```python
from build123d import *

# Parameters (mm, degrees)
SKETCH1_R           = 1.355900406
BOSS_EXTRUDE1_DEPTH = 1.5875
SKETCH3_R           = 1.524
CUT_EXTRUDE1_DEPTH  = 2.5875
SKETCH5_W           = 2.0955
SKETCH5_H           = 13.208
BOSS_EXTRUDE3_DEPTH = 1.5875
CUT_EXTRUDE2_DEPTH  = 2.5875
SKETCH8_R           = 2.4257
CUT_EXTRUDE3_DEPTH  = 2.5875


with BuildPart() as part:
    # Sketch1 → Boss-Extrude1 (new body)
    with BuildSketch(Plane.XY):
        with BuildLine():
            Line((-301.9473, 111.74645), (-305.87795, 115.6771))
            Line((-305.87795, 115.6771), (-316.1078, 115.6771))
            Line((-316.1078, 115.6771), (-316.1078, 128.8851))
            Line((-316.1078, 128.8851), (-305.87795, 128.8851))
            Line((-305.87795, 128.8851), (-301.9473, 132.81575))
            Line((-301.9473, 132.81575), (-301.9473, 150.9704))
            ThreePointArc((-301.9473, 150.9704), (-303.063223164, 153.664476836), (-305.7573, 154.7804))
            Line((-305.7573, 154.7804), (-397.247125, 154.7804))
            ThreePointArc((-397.247125, 154.7804), (-399.946077222, 153.659592612), (-401.0571, 150.956597849))
            Line((-401.0571, 150.956597849), (-401.0571, 148.341))
            Line((-401.0571, 148.341), (-399.1521, 148.341))
            Line((-399.1521, 148.341), (-399.1521, 95.6449))
            Line((-399.1521, 95.6449), (-401.0571, 95.6449))
            Line((-401.0571, 95.6449), (-401.0571, 91.659304166))
            ThreePointArc((-401.0571, 91.659304166), (-399.951018769, 88.947400452), (-397.2472, 87.8217))
            Line((-397.2472, 87.8217), (-378.5565, 87.8217))
            Line((-378.5565, 87.8217), (-368.3165, 91.1883))
            Line((-368.3165, 91.1883), (-315.9973, 91.1883))
            Line((-315.9973, 91.1883), (-305.7573, 87.8217))
            ThreePointArc((-305.7573, 87.8217), (-303.063223164, 88.937623164), (-301.9473, 91.6317))
            Line((-301.9473, 91.6317), (-301.9473, 111.74645))
        make_face()
        with Locations((-305.7573, 91.6317)):
            Circle(SKETCH1_R, mode=Mode.SUBTRACT)
        with Locations((-305.7573, 150.9704)):
            Circle(SKETCH1_R, mode=Mode.SUBTRACT)
        with Locations((-397.247125, 150.9704)):
            Circle(SKETCH1_R, mode=Mode.SUBTRACT)
        with Locations((-397.2472, 91.6317)):
            Circle(SKETCH1_R, mode=Mode.SUBTRACT)
    extrude(amount=BOSS_EXTRUDE1_DEPTH)

    # Sketch3 → Cut-Extrude1 (cut, through all)
    with BuildSketch(Plane.XY.offset(1.5875)):
        with Locations((-397.247125, 150.9704)):
            Circle(SKETCH3_R)
        with Locations((-305.7573, 150.9704)):
            Circle(SKETCH3_R)
        with Locations((-305.7573, 91.6317)):
            Circle(SKETCH3_R)
        with Locations((-397.2472, 91.6317)):
            Circle(SKETCH3_R)
    extrude(amount=-CUT_EXTRUDE1_DEPTH, mode=Mode.SUBTRACT)

    # Sketch5 → Boss-Extrude3 (add)
    with BuildSketch(Plane.XY.offset(1.5875)):
        with Locations((-315.06005, 122.2811)):
            Rectangle(SKETCH5_W, SKETCH5_H)
    extrude(amount=-BOSS_EXTRUDE3_DEPTH)

    # Sketch4 → Cut-Extrude2 (cut, through all)
    with BuildSketch(Plane.XY.offset(1.5875)):
        Polygon((-301.9473, 133.571034757), (-305.87795, 129.6471), (-314.0123, 129.6471), (-314.0123, 113.6451), (-305.87795, 113.6451), (-301.9473, 109.71445), align=None)
    extrude(amount=-CUT_EXTRUDE2_DEPTH, mode=Mode.SUBTRACT)

    # Sketch8 → Cut-Extrude3 (cut, through all)
    with BuildSketch(Plane.XY.offset(1.5875)):
        with Locations((-363.6180125, 150.7799)):
            Circle(SKETCH8_R)
        with Locations((-355.5408125, 150.7799)):
            Circle(SKETCH8_R)
        with Locations((-347.4636125, 150.7799)):
            Circle(SKETCH8_R)
        with Locations((-339.3864125, 150.7799)):
            Circle(SKETCH8_R)
        with Locations((-339.3864125, 142.7027)):
            Circle(SKETCH8_R)
        with Locations((-347.4636125, 142.7027)):
            Circle(SKETCH8_R)
        with Locations((-355.5408125, 142.7027)):
            Circle(SKETCH8_R)
        with Locations((-363.6180125, 142.7027)):
            Circle(SKETCH8_R)
        with Locations((-363.6180125, 95.1888)):
            Circle(SKETCH8_R)
        with Locations((-339.3864125, 95.1888)):
            Circle(SKETCH8_R)
        with Locations((-347.4636125, 95.1888)):
            Circle(SKETCH8_R)
        with Locations((-355.5408125, 95.1888)):
            Circle(SKETCH8_R)
        with Locations((-363.6180125, 103.266)):
            Circle(SKETCH8_R)
        with Locations((-355.5408125, 103.266)):
            Circle(SKETCH8_R)
        with Locations((-347.4636125, 103.266)):
            Circle(SKETCH8_R)
        with Locations((-339.3864125, 103.266)):
            Circle(SKETCH8_R)
    extrude(amount=-CUT_EXTRUDE3_DEPTH, mode=Mode.SUBTRACT)


solid = part.part
```
The model under review builds one solid part; all positions refer to its coordinate system, in mm. A direction names the side the tool comes from. Round coordinates to 2 decimals unless told otherwise and drop trailing zeros. Loops run counter-clockwise (first coordinate to the right, second up) from the corner with the lowest first, then second, coordinate; pieces in that order, holes last.
1) Consider section A-A on x = -339. State the section outline as (y, z) points, then the cut area to 3 significant figures.
Values follow:
outline: (91.19, 0) - (92.79, 0) - (92.79, 1.59) - (91.19, 1.59) - close; (97.58, 0) - (100.87, 0) - (100.87, 1.59) - (97.58, 1.59) - close; (105.66, 0) - (140.31, 0) - (140.31, 1.59) - (105.66, 1.59) - close; (145.1, 0) - (148.39, 0) - (148.39, 1.59) - (145.1, 1.59) - close; (153.17, 0) - (154.78, 0) - (154.78, 1.59) - (153.17, 1.59) - close
area: 70.5 mm2
2) Consider section B-B on y = 123. State the section outline as (x, z) points.
Values follow:
outline: (-399.15, 0) - (-314.01, 0) - (-314.01, 1.59) - (-399.15, 1.59) - close
3) Clearance check with a flat-ended pin moving along its axis: P1, Ø0.8, axis at x = -400, z = 1, coming from the -Y side. State where the tip first meets the part, or that it passes through.
Values follow:
P1: stops at y = 88.63
4) Consider section D-D on x = -372.5. State the section outline as (y, z) points, then the cut area to 3 significant figures.
Values follow:
outline: (89.81, 0) - (154.78, 0) - (154.78, 1.59) - (89.81, 1.59) - close
area: 103 mm2
5) Wall thickness on line 1 along X through (y, z) = (103.5, 1.55); line 2 along X through (y, z) = (104.5, 1.1); line 3 along X through (y, z) = (99.5, 1): over which ranges is each line inside the solid? List them lowest first.
Values follow:
line 1: x = -399.15 to -366.03, -361.2 to -357.96, -353.13 to -349.88, -345.05 to -341.8, -336.97 to -301.95
line 2: x = -399.15 to -365.71, -361.53 to -357.63, -353.45 to -349.55, -345.38 to -341.47, -337.3 to -301.95
line 3: x = -399.15 to -301.95
6) Consider section C-C on z = 0.55. Give the number of separate pieces and of enclosed holes in the cut face, then the cut area to 3 significant figures.
Values follow:
separate pieces: 1
enclosed holes: 20
area: 5,780 mm2
7) The part is to be moulded in two halves that separate along Y. For faces 4 (the face through (-352, 122, 0)), 5 (the face through (-357.964, 150.887, 0.805)), 6 (the face through (-373.51, 89.48, 0.78)), 7 (the face through (-303, 153.6, 0.8)), say which applies: pulls with the +Y half, pulls with the -Y half, needs draft (parallel to the pull), parting line crosses it, or undercut.
Values follow:
face 4: needs draft
face 5: undercut
face 6: pulls with the -Y half
face 7: pulls with the +Y half
8) Tool access review of faces 1 (the face through (-303.94, 111.707, 0.805)), 2 (the face through (-310.95, 89.53, 0.78)), 3 (the face through (-303, 89, 1)): name each direction out of +Z, -Z, +X, -X, +Y, -Y from which nothing blocks a thin tool from reaching the whole face with its end or side.
Values follow:
face 1: +Z, -Z, +X
face 2: +Z, -Z, -Y
face 3: +Z, -Z, +X, -Y
